```python
from build123d import *

# Parameters (mm, degrees)
F3_R     = 5
F4_DEPTH = 20.001


with BuildPart() as f1:
    # F0 (on Front) → F1 (revolve)
    with BuildSketch(Plane.XZ):
        Polygon((0, 7), (0, 0), (50, 0), (50, 7), (44, 7), (44, 10), (6, 10), (6, 7), align=None)
    revolve(axis=Axis((25, 0, 0), (-1, 0, 0)))

    # F3 (on offset) → F4 (cut, through all)
    with BuildSketch(Plane.XY.offset(10)):
        with Locations((25, 0)):
            Circle(F3_R)
    extrude(amount=-F4_DEPTH, mode=Mode.SUBTRACT)


solid = f1.part
```
The listing builds one solid part. Answer for the finished solid, in the listing's coordinates (mm). A direction names the side the tool comes from. Give positions to 0.01 mm unless a question says otherwise; leave off trailing zeros. Loops run counter-clockwise (first coordinate to the right, second up) from the corner with the lowest first, then second, coordinate; pieces in that order, holes last. Notation, with made-up numbers: (-25.5, -10) - (0.5, -10) arc R11 ccw to (0.5, 9) - close; hole circle Ø2 at (75.25, -5.5). An arc over 180 degrees is marked (long way). Return JSON: item names as keys, results as strings. Group by question number.
1. Find section B-B (y = 0). Write down the section's boundary in (x, z), then the cut area to 3 significant figures.
2. Find section D-D (x = 5.5). Write down the section's boundary in (y, z), then the cut area to 3 significant figures.
3. Which of the six approach directions +Z, -Z, +X, -X, +Y, -Y give full straight-line access (tool end or side, diameter ignored) to faces 4 (the cylindrical face through (46.958, -2.681, 6.466)), 5 (the flat face through (6, 7, 2)), 6 (the flat face through (0, 0, 0))?
4. Straight lines are drawn through the part: line 1 (X direction, y = 0, z = 1); line 2 (X direction, y = -6.25, z = 7.75); line 3 (Y direction, x = 25, z = -5). For each, find the intervals that lie inside material, in ascending order. Write a range as [from, to].
5. Given pin 1 Ø4 at (x, z) = (22, 6.5) entering from +Y; pin 2 Ø3 at (x, y) = (28.5, -2.5) entering from -Z; pin 3 Ø8 at (x, y) = (31, 5.5) entering from +Z, each flat-ended and moving along its own axis, determine where each tip first touches the part or whether it passes through.
6. Find section A-A (z = 0). Write down the section's boundary in (x, y), then the cut area to 3 significant figures.
7. Find section C-C (y = -6). Write down the section's boundary in (x, z), then the cut area to 3 significant figures.
8. Determine the mould class of faces 1 (the cylindrical face through (28, 4, 0)), 2 (the cylindrical face through (24.734, -8.872, 4.614)), 3 (the flat face through (50, 0, 0)) for opening direction Y: pulls with the +Y half, pulls with the -Y half, needs draft (parallel to the pull), parting line crosses it, or undercut.
Verdict:
{
 "1": {"outline": "(0, -7) - (6, -7) - (6, -10) - (20, -10) - (20, 10) - (6, 10) - (6, 7) - (0, 7) - close; (30, -10) - (44, -10) - (44, -7) - (50, -7) - (50, 7) - (44, 7) - (44, 10) - (30, 10) - close", "area": "728 mm^2"},
 "2": {"outline": "circle Ø14 at (0, 0)", "area": "154 mm^2"},
 "3": {"face 4": "+X", "face 5": "-X", "face 6": "+Z, -Z, -X, +Y, -Y"},
 "4": {"line 1": "x = [0, 20], [30, 50]", "line 2": "x = [6, 44]", "line 3": "y = [-8.66, -5], [5, 8.66]"},
 "5": {"pin 1": "stops at y = 8.93", "pin 2": "stops at z = -9.87", "pin 3": "stops at z = 9.89"},
 "6": {"outline": "(0, -7) - (6, -7) - (6, -10) - (44, -10) - (44, -7) - (50, -7) - (50, 7) - (44, 7) - (44, 10) - (6, 10) - (6, 7) - (0, 7) - close; hole circle Ø10 at (25, 0)", "area": "849 mm^2"},
 "7": {"outline": "(0, -3.61) - (6, -3.61) - (6, -8) - (44, -8) - (44, -3.61) - (50, -3.61) - (50, 3.61) - (44, 3.61) - (44, 8) - (6, 8) - (6, 3.61) - (0, 3.61) - close", "area": "695 mm^2"},
 "8": {"face 1": "undercut", "face 2": "parting line crosses it", "face 3": "needs draft"}
}
